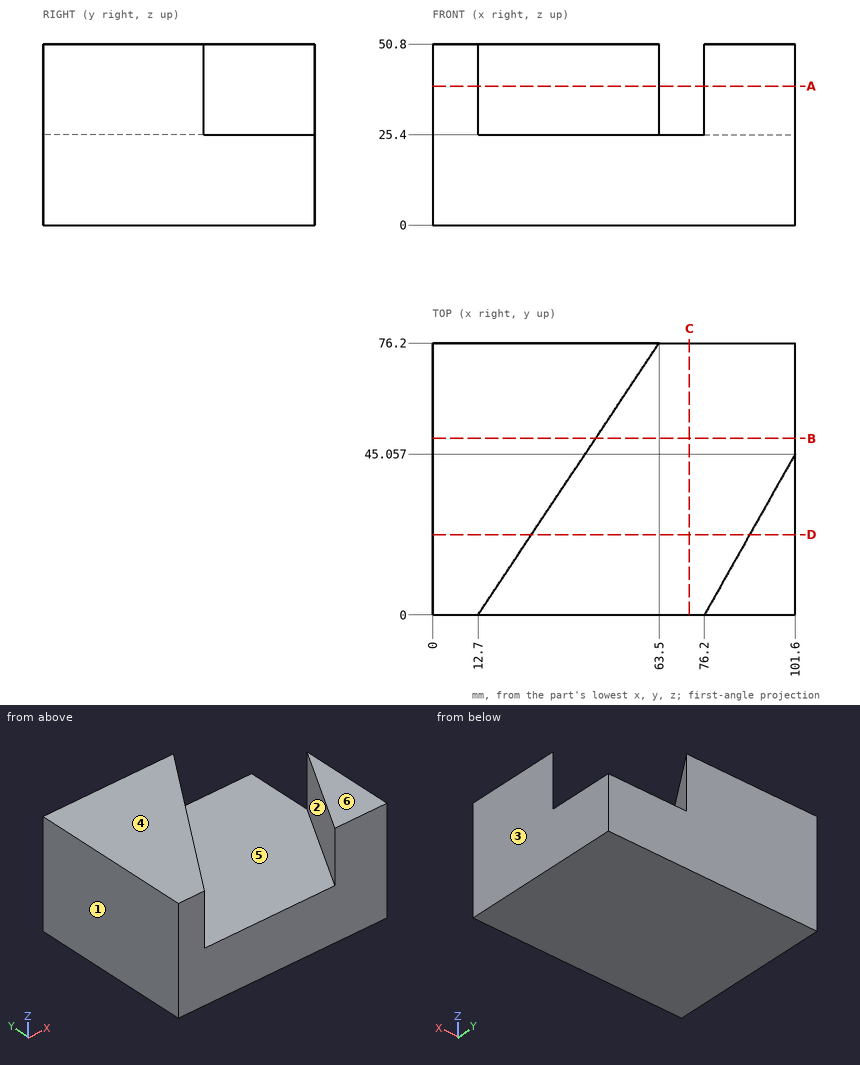
Verification items for this drawing (mm, ordinates from the low corner). A direction names the side the tool comes from. Give positions to 0.01 mm unless a question says otherwise; leave off trailing zeros. Loops run counter-clockwise (first coordinate to the right, second up) from the corner with the lowest first, then second, coordinate; pieces in that order, holes last.
(1) Thickness scan on L1, parallel to Z at x = 72.5, y = 66.5; L2, parallel to X at y = 10.5, z = 29.5; L3, parallel to X at y = 52.5, z = 34. Record the ranges inside material, lowest first.
From the geometry:
L1: z = 0 to 25.4
L2: x = 0 to 19.7, 82.12 to 101.6
L3: x = 0 to 47.7
(2) Section check C-C on x = 72. Record the cut outline in (y, z).
From the geometry:
outline: (0, 0) - (76.2, 0) - (76.2, 25.4) - (0, 25.4) - close
(3) Depth check by flat-ended pin: pin 1 Ø5 at (x, y) = (82, 54.5) entering from -Z; pin 2 Ø23 at (x, y) = (55.5, 35) entering from +Z; pin 3 Ø5 at (x, z) = (30.5, 36.5) entering from -Y. Enter the tip coordinate at first touch or a pass-through.
From the geometry:
pin 1: stops at z = 0
pin 2: stops at z = 25.4
pin 3: stops at y = 22.95
(4) Section check A-A on z = 39. Record the cut outline in (x, y).
From the geometry:
outline: (0, 0) - (12.7, 0) - (63.5, 76.2) - (0, 76.2) - close; (76.2, 0) - (101.6, 0) - (101.6, 45.06) - close
(5) Set-up check for the marked faces 5 and 6: record each of +Z, -Z, +X, -X, +Y, -Y from which the full face is reachable in a straight line by a thin tool's end or side.
From the geometry:
face 5: +Z
face 6: +Z, +X, -X, +Y, -Y
(6) Section check B-B on y = 49.5. Record the cut outline in (x, z), then the cut area to 3 significant figures.
From the geometry:
outline: (0, 0) - (101.6, 0) - (101.6, 25.4) - (45.7, 25.4) - (45.7, 50.8) - (0, 50.8) - close
area: 3,740 mm2
(7) Release check for a two-part mould opening along X. For the marked faces 1, 2, 3 and 4 record: released by +X, released by -X, zero draft, split by the parting line, or undercut.
From the geometry:
face 1: released by -X
face 2: undercut
face 3: released by +X
face 4: zero draft
(8) Section check D-D on y = 22.5. Record the cut outline in (x, z).
From the geometry:
outline: (0, 0) - (101.6, 0) - (101.6, 50.8) - (88.88, 50.8) - (88.88, 25.4) - (27.7, 25.4) - (27.7, 50.8) - (0, 50.8) - close
